Verification items for the finished model (mm, model axes). Round coordinates to 2 decimals unless told otherwise and drop trailing zeros. Order: outer loops, then holes, each group sorted by start corner. A loop starts at its lowest first (then second) coordinate and runs counter-clockwise, first axis right, second up. Notation, with made-up numbers: (-6.5, 86.25) -> (21.5, 86.25) arc R18 cw to (21.5, 121.25) -> close; hole circle Ø7 at (-30.75, 62.25). An arc over 180 degrees is marked (long way). Answer in a Markdown table with one row per item. Add a question column.
```python
from build123d import *

# Parameters (mm, degrees)
ESBO_O1_R                = 2.25
ESBO_O1_R_2              = 1.8
ESBO_O1_W                = 15
ESBO_O1_H                = 6
ESBO_O1_W_2              = 31
ESBO_O1_H_2              = 9
RESSALTO_EXTRUS_O1_DEPTH = 3


with BuildPart() as part:
    # Esboço1 → Ressalto-extrusão1 (new body)
    with BuildSketch(Plane.XY):
        with BuildLine():
            Line((-94, 26.5), (83, 26.5))
            ThreePointArc((83, 26.5), (109.5, 0), (83, -26.5))
            Line((83, -26.5), (-94, -26.5))
            ThreePointArc((-94, -26.5), (-120.5, 0), (-94, 26.5))
        make_face()
        with Locations((-22.5, 0)):
            Circle(ESBO_O1_R, mode=Mode.SUBTRACT)
        with Locations((22.5, 0)):
            Circle(ESBO_O1_R, mode=Mode.SUBTRACT)
        with Locations((-109.1, 0)):
            Circle(ESBO_O1_R_2, mode=Mode.SUBTRACT)
        with Locations((-72.5, 0)):
            Circle(ESBO_O1_R_2, mode=Mode.SUBTRACT)
        with Locations((62.5, 0)):
            Circle(ESBO_O1_R_2, mode=Mode.SUBTRACT)
        with Locations((99.1, 0)):
            Circle(ESBO_O1_R_2, mode=Mode.SUBTRACT)
        Rectangle(ESBO_O1_W, ESBO_O1_H, mode=Mode.SUBTRACT)
        with Locations((-90.8, 0)):
            Rectangle(ESBO_O1_W_2, ESBO_O1_H_2, mode=Mode.SUBTRACT)
        with Locations((80.8, 0)):
            Rectangle(ESBO_O1_W_2, ESBO_O1_H_2, mode=Mode.SUBTRACT)
    extrude(amount=RESSALTO_EXTRUS_O1_DEPTH)


solid = part.part
```
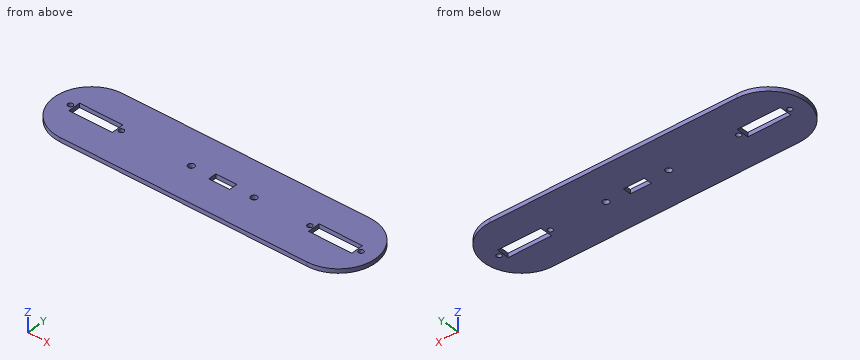
1) Cross-section at B-B, the plane z = 1.55. Give the number of separate pieces and of enclosed holes in the cut face, and give its area (3 significant figures).
2) Depth check by flat-ended pin: P1, Ø1.5, axis at y = 19.5, z = 2.5, coming from the -X side; P2, Ø1, axis at y = -20, z = 1.5, coming from the +X side; P3, Ø0.9, axis at y = 0.5, z = 1, coming from the -X side. Enter the tip coordinate at first touch or a pass-through.
3) Thickness scan on L1, parallel to Y at x = -82, z = 1; L2, parallel to Y at x = 0.5, z = 1.1; L3, parallel to X at y = -2, z = 1.25. Record the ranges inside material, lowest first. Write a range as [from, to].
4) Cross-section at C-C, the plane y = -15. Record the boundary of the cut face in (x, z).
5) Cross-section at A-A, the plane x = 5. Record the boundary of the cut face in (y, z), and give its area (3 significant figures).
Results below:
| question | item | result |
|---|---|---|
| 1 | separate pieces | 1 |
| 1 | enclosed holes | 9 |
| 1 | area | 10,900 mm² |
| 2 | P1 | x = -112.73 |
| 2 | P2 | x = 100.94 |
| 2 | P3 | x = -120.5 |
| 3 | L1 | [-26.5, -4.5], [4.5, 26.5] |
| 3 | L2 | [-26.5, -3], [3, 26.5] |
| 3 | L3 | [-120.42, -106.3], [-75.3, -23.53], [-21.47, -7.5], [7.5, 21.47], [23.53, 65.3], [96.3, 109.42] |
| 4 | outline | (-115.85, 0) -> (104.85, 0) -> (104.85, 3) -> (-115.85, 3) -> close |
| 5 | outline | (-26.5, 0) -> (-3, 0) -> (-3, 3) -> (-26.5, 3) -> close; (3, 0) -> (26.5, 0) -> (26.5, 3) -> (3, 3) -> close |
| 5 | area | 141 mm² |
